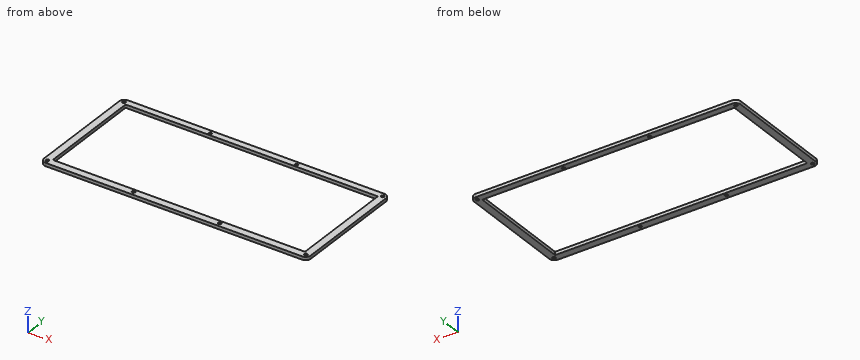
from build123d import *

# Parameters (mm, degrees)
SKETCH_W     = 263.525
SKETCH_H     = 117.475
PAD_DEPTH    = 3.175
SKETCH002_W  = 249.2375
SKETCH002_H  = 103.98125
POCKET_DEPTH = 3.176
SKETCH001_R  = 1.5494
HOLE_DEPTH   = 3.176
FILLET_R     = 5.08
FILLET001_R  = 1.27


with BuildPart() as part:
    # Sketch → Pad (new body)
    with BuildSketch(Plane.XY):
        Rectangle(SKETCH_W, SKETCH_H)
    extrude(amount=PAD_DEPTH)

    # Sketch002 (on Face6 of Pad) → Pocket (cut, through all)
    with BuildSketch(Plane.XY.offset(3.175)):
        with Locations((0, 0.396875)):
            Rectangle(SKETCH002_W, SKETCH002_H)
    extrude(amount=-POCKET_DEPTH, mode=Mode.SUBTRACT)

    # Sketch001 (on Face6 of Pad) → Hole (cut, through all)
    with BuildSketch(Plane.XY.offset(3.175)):
        with Locations((-42.597917, 54.76875)):
            Circle(SKETCH001_R)
        with Locations((42.597917, 54.76875)):
            Circle(SKETCH001_R)
        with Locations((42.597917, -54.76875)):
            Circle(SKETCH001_R)
        with Locations((-42.597917, -54.76875)):
            Circle(SKETCH001_R)
        with Locations((-127.79375, -54.76875)):
            Circle(SKETCH001_R)
        with Locations((-127.79375, 54.76875)):
            Circle(SKETCH001_R)
        with Locations((127.79375, 54.76875)):
            Circle(SKETCH001_R)
        with Locations((127.79375, -54.76875)):
            Circle(SKETCH001_R)
    extrude(amount=-HOLE_DEPTH, mode=Mode.SUBTRACT)

    # Fillet
    fillet_edges = [part.edges().sort_by_distance(p)[0] for p in [
        (-131.7625, 58.7375, 1.5875),
        (-131.7625, -58.7375, 1.5875),
        (131.7625, -58.7375, 1.5875),
        (131.7625, 58.7375, 1.5875),
    ]]
    fillet(fillet_edges, radius=FILLET_R)

    # Fillet001
    fillet001_edges = [part.edges().sort_by_distance(p)[0] for p in [
        (-124.61875, -51.59375, 1.5875),
        (-41.048517, 54.76875, 1.5875),
        (-126.24435, 54.76875, 1.5875),
        (-124.61875, 52.3875, 1.5875),
    ]]
    fillet(fillet001_edges, radius=FILLET001_R)


solid = part.part
Here's how the part is built. I have some questions about the finished solid (model axes, mm). Give positions to 0.01 mm unless a question says otherwise; leave off trailing zeros. Order: outer loops, then holes, each group sorted by start corner. A loop starts at its lowest first (then second) coordinate and runs counter-clockwise, first axis right, second up. Notation, with made-up numbers: M 6,-14 L 63,-14 A16 ccw 63,-1 Z; hole C 25,29 d5. An arc over 180 degrees is marked long. Answer as a JSON object with one key per item and string values. Group by question number.
1) Suppose I cut it at A-A, the plane y = -42.5. Write out the boundary of the cut face in (x, z) (1 decimal).
2) Suppose I cut it at B-B, the plane x = 97.5. Write out the boundary of the cut face in (y, z) (1 decimal).
3) Please list where these lines run through material, in increasing order: L1, parallel to X at y = 15, z = 2.7; L2, parallel to Y at x = 43, z = 2.1; L3, parallel to Y at x = -35.5, z = 1.95. Write a range as [from, to].
4) Suppose I cut it at C-C, the plane z = 0.7. Count the separate pieces of the cut face and the enclosed holes in it, plus the area to 3 significant figures.
Results found:
{
 "1": {"outline": "M -131.8,0 L -124.6,0 L -124.6,3.2 L -131.8,3.2 Z; M 124.6,0 L 131.8,0 L 131.8,3.2 L 124.6,3.2 Z"},
 "2": {"outline": "M -58.7,0 L -51.6,0 L -51.6,3.2 L -58.7,3.2 Z; M 52.4,0 L 58.7,0 L 58.7,3.2 L 52.4,3.2 Z"},
 "3": {"L1": "[-131.76, -124.62], [124.62, 131.76]", "L2": "[-58.74, -56.27], [-53.27, -51.59], [52.39, 53.27], [56.27, 58.74]", "L3": "[-58.74, -51.59], [52.39, 58.74]"},
 "4": {"separate pieces": "1", "enclosed holes": "9", "area": "4,960 mm²"}
}
